```python
from build123d import *

# Parameters (mm, degrees)
BOSS_EXTRUDE1_DEPTH            = 38.1
BOSS_EXTRUDE3_DEPTH            = 76.2
CUT_EXTRUDE1_REACH             = 53.888
SKETCH4_R                      = 3.175
CUT_EXTRUDE1_DIRECTION_2_DEPTH = 6.35
CUT_EXTRUDE2_REACH             = 56.243
SKETCH5_R                      = 1.5875


with BuildPart() as part:
    # Sketch1 → Boss-Extrude1 (new, symmetric)
    with BuildSketch(Plane.XY):
        with BuildLine():
            Line((12.7, 12.7), (-12.7, 12.7))
            Line((-12.7, 12.7), (-12.7, 2.921))
            Line((-12.7, 2.921), (-10.16, 2.921))
            Line((-10.16, 2.921), (-10.16, 5.585607176))
            ThreePointArc((-10.16, 5.585607176), (-9.787392339, 6.163859076), (-9.106849574, 6.063493377))
            Line((-9.106849574, 6.063493377), (-5.08, 2.54))
            Line((-5.08, 2.54), (-5.08, -2.54))
            Line((-5.08, -2.54), (-9.106849574, -6.063493377))
            ThreePointArc((-9.106849574, -6.063493377), (-9.787392339, -6.163859076), (-10.16, -5.585607176))
            Line((-10.16, -5.585607176), (-10.16, -2.921))
            Line((-10.16, -2.921), (-12.7, -2.921))
            Line((-12.7, -2.921), (-12.7, -12.7))
            Line((-12.7, -12.7), (-8.89, -12.7))
            Line((-8.89, -12.7), (-8.89, -13.97))
            Line((-8.89, -13.97), (-15.24, -13.97))
            Line((-15.24, -13.97), (-15.24, 15.24))
            Line((-15.24, 15.24), (15.24, 15.24))
            Line((15.24, 15.24), (15.24, -13.97))
            Line((15.24, -13.97), (8.89, -13.97))
            Line((8.89, -13.97), (8.89, -12.7))
            Line((8.89, -12.7), (12.7, -12.7))
            Line((12.7, -12.7), (12.7, -2.921))
            Line((12.7, -2.921), (10.16, -2.921))
            Line((10.16, -2.921), (10.16, -5.585607176))
            ThreePointArc((10.16, -5.585607176), (9.787392339, -6.163859076), (9.106849574, -6.063493377))
            Line((9.106849574, -6.063493377), (5.08, -2.54))
            Line((5.08, -2.54), (5.08, 2.54))
            Line((5.08, 2.54), (9.106849574, 6.063493377))
            ThreePointArc((9.106849574, 6.063493377), (9.787392339, 6.163859076), (10.16, 5.585607176))
            Line((10.16, 5.585607176), (10.16, 2.921))
            Line((10.16, 2.921), (12.7, 2.921))
            Line((12.7, 2.921), (12.7, 12.7))
        make_face()
    extrude(amount=BOSS_EXTRUDE1_DEPTH, both=True)

    # Sketch6 → Boss-Extrude3 (add)
    with BuildSketch(Plane(origin=(0, 0, -38.1), x_dir=(-1, 0, 0), z_dir=(0, 0, -1))):
        with BuildLine():
            Line((-15.24, 15.24), (-31.115, 15.24))
            Line((-31.115, 15.24), (-31.115, 12.7))
            ThreePointArc((-31.115, 12.7), (-20.774098647, 0.795596044), (-15.24, -13.97))
            Line((-15.24, -13.97), (-15.24, 15.24))
        make_face()
        with BuildLine():
            Line((15.24, 15.24), (31.115, 15.24))
            Line((31.115, 15.24), (31.115, 12.7))
            ThreePointArc((31.115, 12.7), (20.774098647, 0.795596044), (15.24, -13.97))
            Line((15.24, -13.97), (15.24, 15.24))
        make_face()
    extrude(amount=-BOSS_EXTRUDE3_DEPTH)

    # Sketch4 → Cut-Extrude1 (cut, up to next)
    with BuildSketch(Plane(origin=(0, 2.54, 0), x_dir=(1, 0, 0), z_dir=(0, 1, 0)), mode=Mode.PRIVATE) as cut_extrude1_sk1:
        with Locations(Location((23.495, 0, 0), (0, 0, 90))):
            Circle(SKETCH4_R)
    cut_extrude1_tool1 = extrude(cut_extrude1_sk1.sketch, amount=-CUT_EXTRUDE1_REACH, mode=Mode.PRIVATE) & part.part
    cut_extrude1 = cut_extrude1_tool1.solids().sort_by_distance((23.495, 2.54, 0))[0]
    add(cut_extrude1, mode=Mode.SUBTRACT)

    # Sketch4 → Cut-Extrude1 direction 2 (cut)
    with BuildSketch(Plane(origin=(0, 2.54, 0), x_dir=(1, 0, 0), z_dir=(0, 1, 0))):
        with Locations(Location((23.495, 0, 0), (0, 0, 90))):
            Circle(SKETCH4_R)
    cut_extrude1_direction_2 = extrude(amount=CUT_EXTRUDE1_DIRECTION_2_DEPTH, mode=Mode.SUBTRACT)

    # Sketch5 → Cut-Extrude2 (cut, up to next)
    with BuildSketch(Plane.XZ.offset(-8.89), mode=Mode.PRIVATE) as cut_extrude2_sk1:
        with Locations(Location((23.495, 0, 0), (0, 0, 270))):
            Circle(SKETCH5_R)
    cut_extrude2_tool1 = extrude(cut_extrude2_sk1.sketch, amount=-CUT_EXTRUDE2_REACH, mode=Mode.PRIVATE) & part.part
    cut_extrude2 = cut_extrude2_tool1.solids().sort_by_distance((23.495, 8.89, 0))[0]
    add(cut_extrude2, mode=Mode.SUBTRACT)

    # Mirror1: Cut-Extrude1, Cut-Extrude1 direction 2, Cut-Extrude2 across plane
    add(cut_extrude1.mirror(Plane(origin=(0, 0, 0), x_dir=(0, 0, 1), z_dir=(1, 0, 0))), mode=Mode.SUBTRACT)
    add(cut_extrude1_direction_2.mirror(Plane(origin=(0, 0, 0), x_dir=(0, 0, 1), z_dir=(1, 0, 0))), mode=Mode.SUBTRACT)
    add(cut_extrude2.mirror(Plane(origin=(0, 0, 0), x_dir=(0, 0, 1), z_dir=(1, 0, 0))), mode=Mode.SUBTRACT)


solid = part.part
```
Read the model definition and answer for the solid it produces. Units are mm, in the model's axes. A direction names the side the tool comes from. Give positions to 0.01 mm unless a question says otherwise; leave off trailing zeros. Order: outer loops, then holes, each group sorted by start corner. A loop starts at its lowest first (then second) coordinate and runs counter-clockwise, first axis right, second up.
(1) Given pin 1 (12.5 mm diameter, centred on x = 3.5, z = -4, fed in from -Y); pin 2 (4 mm diameter, centred on y = -1, z = 2, fed in from +X); pin 3 (6 mm diameter, centred on y = -6, z = 16.5, fed in from -X); pin 4 (1 mm diameter, centred on y = -7.5, z = 18.5, fed in from +X), each flat-ended and moving along its own axis, determine where each tip first touches the part or whether it passes through.
(2) For a pull along X with two mould halves and no side action, classify faces 1 (the cylindrical face through (-19.193, -2.101, -0.533)), 2 (the flat face through (7, 4, -38.1)), 3 (the cylindrical face through (20.347, 5.501, 0.413)) as released by +X, released by -X, zero draft, split by the parting line, or undercut.
(3) For faces 4 (the flat face through (7, 4, 38.1)), 5 (the flat face through (0, 12.7, 1)), 6 (the flat face through (-22, 8.89, -1)), determine the directions among +Z, -Z, +X, -X, +Y, -Y from which every point of the face is accessible in a straight line to the end or side of a thin tool.
(4) Find section A-A (y = 1). Give the vertices of the cut face in (x, z) (3 decimals).
(5) Find section C-C (x = 8). Give the vertices of the cut face in (y, z) (3 decimals).
(6) Find section D-D (y = -4.5). Give the vertices of the cut face in (x, z), plus the area to 3 significant figures.
(7) Straight lines are drawn through the part: L1, parallel to X at y = 12.75, z = 0 (1 decimal); L2, parallel to Y at x = 10.5, z = -5; L3, parallel to Y at x = 10, z = -25. For each, find the intervals that lie inside material, in ascending order.
Result sheet:
1. pin 1: stops at y = -13.97
1. pin 2: stops at x = 20.9
1. pin 3: stops at x = -18.76
1. pin 4: stops at x = 17.11
2. face 1: released by -X
2. face 2: zero draft
2. face 3: undercut
3. face 4: +Z, +X, -X, +Y, -Y
3. face 5: +Z, -Z
3. face 6: -Y
4. outline: (-20.897, -38.1) - (-5.08, -38.1) - (-5.08, 38.1) - (-20.897, 38.1) - (-20.897, 1.824) arc R3.175 cw to (-20.897, -1.824) - close; (5.08, -38.1) - (20.897, -38.1) - (20.897, -1.824) arc R3.175 cw to (20.897, 1.824) - (20.897, 38.1) - (5.08, 38.1) - close
5. outline: (-5.095, -38.1) - (5.095, -38.1) - (5.095, 38.1) - (-5.095, 38.1) - close; (12.7, -38.1) - (15.24, -38.1) - (15.24, 38.1) - (12.7, 38.1) - close
6. outline: (-18.08, -38.1) - (-12.7, -38.1) - (-12.7, 38.1) - (-18.08, 38.1) - close; (-10.16, -38.1) - (-7.32, -38.1) - (-7.32, 38.1) - (-10.16, 38.1) - close; (7.32, -38.1) - (10.16, -38.1) - (10.16, 38.1) - (7.32, 38.1) - close; (12.7, -38.1) - (18.08, -38.1) - (18.08, 38.1) - (12.7, 38.1) - close
6. area: 1,250 mm2
7. L1: x = -31.1 to -25.1, -21.9 to 21.9, 25.1 to 31.1
7. L2: y = -13.97 to -12.7, -2.92 to 2.92, 12.7 to 15.24
7. L3: y = -13.97 to -12.7, -6.01 to 6.01, 12.7 to 15.24
